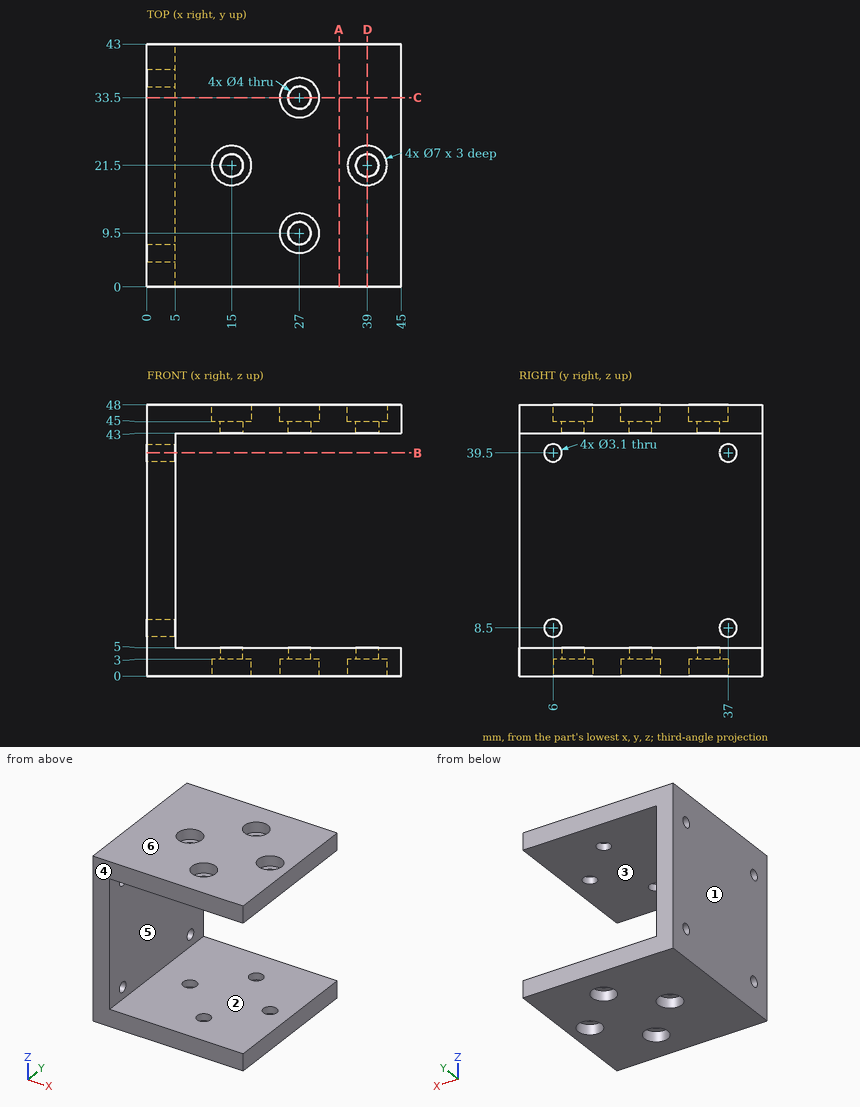
Geometry check sheet. Reference: drawing and pictorial views, mm from the part's lowest x, y, z. A direction names the side the tool comes from. Give positions to 0.01 mm unless a question says otherwise; leave off trailing zeros. Order: outer loops, then holes, each group sorted by start corner. A loop starts at its lowest first (then second) coordinate and runs counter-clockwise, first axis right, second up. Notation, with made-up numbers: M 19.25,60 L 55.25,60 A26 ccw 55.25,90 Z; hole C 25,7 d3. An arc over 180 degrees is marked long. Answer as a JSON object with one key per item and string values. Group by question number.
1) Cross-section at B-B (z = 39.5). Enter the section's corners in (x, y).
2) Cross-section at D-D (x = 39). Enter the section's corners in (y, z), then the cut area to 3 significant figures.
3) Access from +Z, -Z, +X, -X, +Y, -Y to the whole of each face (thin tool, end or side, straight path). Record for the marked faces 1 and 2.
4) Depth check by flat-ended pin: pin 1 Ø1.5 at (y, z) = (22.5, 39) entering from +X; pin 2 Ø7.5 at (x, y) = (39, 20.5) entering from +Z; pin 3 Ø5 at (x, y) = (27, 33.5) entering from -Z; pin 4 Ø5 at (x, y) = (27, 9.5) entering from +Z. Enter the tip coordinate at first touch or a pass-through.
5) Mould release check, pull along Z, two halves, no side actions. Record for the marked faces 3, 4, 5 and 6: released by +Z, released by -Z, zero draft, split by the parting line, or undercut.
6) Cross-section at A-A (x = 34). Enter the section's corners in (y, z).
7) Scan lines: line 1 along Y through (x, z) = (2.75, 39.5); line 2 along Z through (x, y) = (11.5, 10); line 3 along Y through (x, z) = (27, 43.45). Record each from-to range of solid material in increasing order. Write a range as [from, to].
8) Cross-section at C-C (y = 33.5). Enter the section's corners in (x, z).
Result sheet:
{
 "1": {"outline": "M 0,0 L 5,0 L 5,4.45 L 0,4.45 Z; M 0,7.55 L 5,7.55 L 5,35.45 L 0,35.45 Z; M 0,38.55 L 5,38.55 L 5,43 L 0,43 Z"},
 "2": {"outline": "M 0,0 L 18,0 L 18,3 L 19.5,3 L 19.5,5 L 0,5 Z; M 0,43 L 19.5,43 L 19.5,45 L 18,45 L 18,48 L 0,48 Z; M 23.5,3 L 25,3 L 25,0 L 43,0 L 43,5 L 23.5,5 Z; M 23.5,43 L 43,43 L 43,48 L 25,48 L 25,45 L 23.5,45 Z", "area": "372 mm2"},
 "3": {"face 1": "+Z, -Z, -X, +Y, -Y", "face 2": "+X, +Y, -Y"},
 "4": {"pin 1": "stops at x = 5", "pin 2": "stops at z = 48", "pin 3": "stops at z = 3", "pin 4": "stops at z = 45"},
 "5": {"face 3": "undercut", "face 4": "zero draft", "face 5": "undercut", "face 6": "released by +Z"},
 "6": {"outline": "M 0,0 L 43,0 L 43,5 L 0,5 Z; M 0,43 L 43,43 L 43,48 L 0,48 Z"},
 "7": {"line 1": "y = [0, 4.45], [7.55, 35.45], [38.55, 43]", "line 2": "z = [0, 5], [43, 48]", "line 3": "y = [0, 7.5], [11.5, 31.5], [35.5, 43]"},
 "8": {"outline": "M 0,0 L 23.5,0 L 23.5,3 L 25,3 L 25,5 L 5,5 L 5,43 L 25,43 L 25,45 L 23.5,45 L 23.5,48 L 0,48 Z; M 29,3 L 30.5,3 L 30.5,0 L 45,0 L 45,5 L 29,5 Z; M 29,43 L 45,43 L 45,48 L 30.5,48 L 30.5,45 L 29,45 Z"}
}
